The listing builds one solid part. Answer for the finished solid, in the listing's coordinates (mm). Give positions to 0.01 mm unless a question says otherwise; leave off trailing zeros. Write each loop counter-clockwise with the first axis right and the second up, starting at its lowest first coordinate (ties: lowest second). Pieces come first, ordered by that corner, then holes. Notation, with made-up numbers: (61.5, 2.5) - (107.5, 2.5) arc R18 ccw to (107.5, 31.5) - close; hole circle Ø5 at (28.25, 24.25). An arc over 180 degrees is marked (long way). One line per question, with ' | ' between items. Start each with the question number.
1. A cutting plane is placed at A-A (y = -1.25). Determine the outline of the cut face in (x, z), then the cut area to 4 significant figures.
2. Find the intervals of material crossed by L1, parallel to Y at x = -2.75, z = 5.25; L2, parallel to X at y = 1.75, z = 0.75; L3, parallel to Z at x = -3.5, y = -2.5, in increasing order. Write a range as from..to.
3. Given P1, Ø1.5, axis at x = -2, z = 2.5, coming from the +Y side, flat-ended and moving along its own axis, determine where the tip first touches the part or whether it passes through.
```python
from build123d import *

# Parameters (mm, degrees)
SKETCH1_R               = 4
BOSS_EXTRUDE1_DEPTH     = 3.2
SKETCH9_OUTSIDE_W       = 19.044
SKETCH9_OUTSIDE_H       = 21.04
SKETCH9_OUTSIDE_R       = 5.723909236
CUT_EXTRUDE3_DEPTH      = 0.64
SKETCH5_OUTSIDE_W       = 62.042
SKETCH5_OUTSIDE_H       = 64.038
SKETCH5_OUTSIDE_R       = 6.45
CUT_EXTRUDE2_DEPTH      = 12.412716592
CUT_EXTRUDE2_DRAFT      = -60
MIRROR1_COPY_1_SKETCH_W = 62.042
MIRROR1_COPY_1_SKETCH_H = 64.038
MIRROR1_COPY_1_SKETCH_R = 6.45
MIRROR1_COPY_1_DEPTH    = 12.412716592
MIRROR1_COPY_1_DRAFT    = -60


with BuildPart() as part:
    # Sketch1 → Boss-Extrude1 (new, symmetric)
    with BuildSketch(Plane(origin=(0, 0, 0), x_dir=(1, 0, 0), z_dir=(0, 1, 0))):
        Polygon((-6.45, 3.723909236), (-6.45, -3.723909236), (0, -7.447818473), (6.45, -3.723909236), (6.45, 3.723909236), (0, 7.447818473), align=None)
        with Locations(Location((0, 0, 0), (0, 0, 270))):
            Circle(SKETCH1_R, mode=Mode.SUBTRACT)
    extrude(amount=BOSS_EXTRUDE1_DEPTH, both=True)

    # Sketch9 outside → Cut-Extrude3 (cut)
    with BuildSketch(Plane(origin=(0, 3.2, 0), x_dir=(1, 0, 0), z_dir=(0, 1, 0))):
        Rectangle(SKETCH9_OUTSIDE_W, SKETCH9_OUTSIDE_H)
        with Locations(Location((0, 0, 0), (0, 0, 270))):
            Circle(SKETCH9_OUTSIDE_R, mode=Mode.SUBTRACT)
    extrude(amount=-CUT_EXTRUDE3_DEPTH, mode=Mode.SUBTRACT)


with BuildPart() as cut_extrude2_tool:
    # Sketch5 outside → Cut-Extrude2 (with draft: the straight prism first)
    with BuildSketch(Plane(origin=(0, 2.56, 0), x_dir=(1, 0, 0), z_dir=(0, 1, 0))):
        Rectangle(SKETCH5_OUTSIDE_W, SKETCH5_OUTSIDE_H)
        Circle(SKETCH5_OUTSIDE_R, mode=Mode.SUBTRACT)
    extrude(amount=-CUT_EXTRUDE2_DEPTH)
    # Cut-Extrude2: the draft: its side faces are tilted about the plane it starts from
    cut_extrude2_sides = [cut_extrude2_tool.faces().sort_by_distance(p)[0] for p in [
        (0, -3.646358296, 32.019),
        (31.021, -3.646358296, 0),
        (0, -3.646358296, -32.019),
        (-31.021, -3.646358296, 0),
        (-6.45, -3.646358296, 0),
    ]]
    draft(cut_extrude2_sides, Plane(origin=(0, 2.56, 0), x_dir=(1, 0, 0), z_dir=(0, 1, 0)), CUT_EXTRUDE2_DRAFT)


with BuildPart() as part_1:
    add(part.part)

    # Cut-Extrude2: cut by cut_extrude2_tool
    add(cut_extrude2_tool.part, mode=Mode.SUBTRACT)


with BuildPart() as mirror1_copy_1_tool:
    # Mirror1 copy 1 sketch → Mirror1 copy 1 (with draft: the straight prism first)
    with BuildSketch(Plane.XZ.offset(3.2)):
        Rectangle(MIRROR1_COPY_1_SKETCH_W, MIRROR1_COPY_1_SKETCH_H)
        Circle(MIRROR1_COPY_1_SKETCH_R, mode=Mode.SUBTRACT)
    extrude(amount=-MIRROR1_COPY_1_DEPTH)
    # Mirror1 copy 1: the draft: its side faces are tilted about the plane it starts from
    mirror1_copy_1_sides = [mirror1_copy_1_tool.faces().sort_by_distance(p)[0] for p in [
        (0, 3.006358296, 32.019),
        (31.021, 3.006358296, 0),
        (0, 3.006358296, -32.019),
        (-31.021, 3.006358296, 0),
        (-6.45, 3.006358296, 0),
    ]]
    draft(mirror1_copy_1_sides, Plane.XZ.offset(3.2), MIRROR1_COPY_1_DRAFT)


with BuildPart() as part_2:
    add(part_1.part)

    # Mirror1 copy 1: cut by mirror1_copy_1_tool
    add(mirror1_copy_1_tool.part, mode=Mode.SUBTRACT)


solid = part_2.part
```
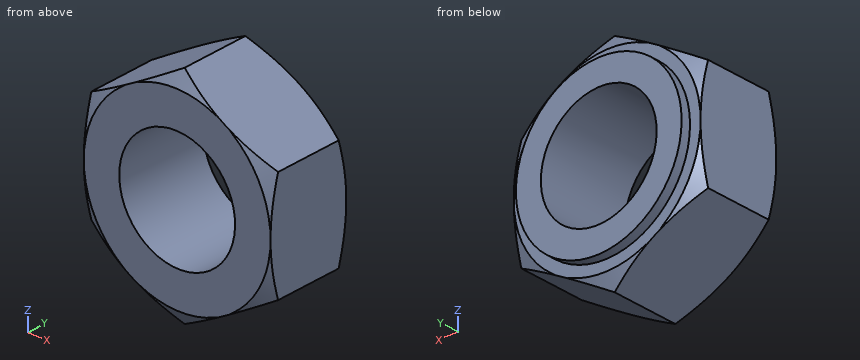
Determined:
1) outline: (-6.45, -3.72) - (0, -7.45) - (6.45, -3.72) - (6.45, 3.72) - (0, 7.45) - (-6.45, 3.72) - close; hole circle Ø8 at (0, 0) | area: 93.85 mm2
2) L1: -3.2..2.56 | L2: -6.45..-3.93, 3.93..6.45 | L3: -5.43..-1.94, 1.94..5.43
3) P1: through
